Can you work these out from the model? Positions are in its coordinate system, mm. A direction names the side the tool comes from. Round coordinates to 2 decimals unless told otherwise and drop trailing zeros. Order: outer loops, then holes, each group sorted by start corner. A loop starts at its lowest first (then second) coordinate and runs counter-clockwise, first axis right, second up.
Q1. If we section it at D-D (z = 1.5): Please give me the cut outline in (x, y).
Q2. Will these pins go through, and if not, where does the flat tip stop? P1, Ø4, axis at x = 6.5, z = 4, coming from the -Y side; P2, Ø4, axis at x = 2.5, z = 17, coming from the -Y side; P3, Ø1.5, axis at x = -7, y = 8.5, coming from the -Z side.
Q3. We'd pull the mould along X, two halves only. Please class faces 3 (the face through (0, 0, 0)), 4 (the face through (-1.5, 11.4, 10.9)), 5 (the face through (0, 0, 4.3)): pulls with the +X half, pulls with the -X half, needs draft (parallel to the pull), parting line crosses it, or undercut.
Q4. For faces 1 (the face through (5, -2, 20)), 2 (the face through (-0.86, -3.88, 11.75)), which set-ups out of +Z, -Z, +X, -X, +Y, -Y let a thin tool reach every point of the face, with its end or its side?
Q5. If I drill on line 1 (Y direction, x = 0, z = 14.75) (3 decimals); line 2 (Y direction, x = 0, z = 4); line 3 (X direction, y = 1.75, z = 13), over which ranges is the centre line in solid material (lowest first)?
Q6. If we section it at B-B (x = 0): Please give me the cut outline in (y, z) (3 decimals), plus the area to 3 significant figures.
Q7. If we section it at A-A (z = 16): Please give me the cut outline in (x, y) (3 decimals).
from build123d import *

# Parameters (mm, degrees)
F0_R     = 11.5
F0_R_2   = 3.985
F1_DEPTH = 20
F2_R     = 3.975
F3_DEPTH = 15.7
F4_SIZE  = 3
F5_SIZE  = 1


with BuildPart() as f1:
    # F0 (on Top) → F1 (new body)
    with BuildSketch(Plane.XY):
        Circle(F0_R)
        Circle(F0_R_2, mode=Mode.SUBTRACT)
        Circle(F0_R_2)
    extrude(amount=F1_DEPTH)

    # F2 (on face) → F3 (cut)
    with BuildSketch(Plane.XY.offset(20)):
        Circle(F2_R)
    extrude(amount=-F3_DEPTH, mode=Mode.SUBTRACT)

    # F4
    f4_edges = [f1.edges().sort_by_distance(p)[0] for p in [
        (-11.5, 0, 0),
    ]]
    chamfer(f4_edges, length=F4_SIZE)

    # F5
    f5_edges = [f1.edges().sort_by_distance(p)[0] for p in [
        (-11.5, 0, 20),
        (-3.975, 0, 20),
    ]]
    chamfer(f5_edges, length=F5_SIZE)


solid = f1.part
Solution:
1. outline: circle Ø20 at (0, 0)
2. P1: stops at y = -10.58
2. P2: stops at y = -11.49
2. P3: stops at z = 1.76
3. face 3: needs draft
3. face 4: parting line crosses it
3. face 5: undercut
4. face 1: +Z, +X, -X, +Y, -Y
4. face 2: +Z
5. line 1: y = -11.5 to -3.975, 3.975 to 11.5
5. line 2: y = -11.5 to 11.5
5. line 3: x = -11.37 to -3.57, 3.57 to 11.37
6. outline: (-11.5, 3) - (-8.5, 0) - (8.5, 0) - (11.5, 3) - (11.5, 19) - (10.5, 20) - (4.975, 20) - (3.975, 19) - (3.975, 4.3) - (-3.975, 4.3) - (-3.975, 19) - (-4.975, 20) - (-10.5, 20) - (-11.5, 19) - close
6. area: 324 mm2
7. outline: circle Ø23 at (0, 0); hole circle Ø7.95 at (0, 0)
